from build123d import *

# Parameters (mm, degrees)
F0_R     = 4.1
F1_DEPTH = 10
F2_R     = 10
F3_R     = 2


with BuildPart() as f1:
    # F0 (on Top) → F1 (new body)
    with BuildSketch(Plane.XY):
        Polygon((70, 30), (70, 40), (70, 50), (-8.4782754802, 92.5), (-30, 92.5), (-30, 67.5), (-10, 67.5), (-10, 12.5), (-30, 12.5), (-30, -12.5), (-8.4782754802, -12.5), align=None)
        with Locations((-20, 0)):
            Circle(F0_R, mode=Mode.SUBTRACT)
        with Locations((-20, 80)):
            Circle(F0_R, mode=Mode.SUBTRACT)
        with BuildLine():
            Line((2, 73.1787940384), (52.0543567222, 46.0717998075))
            ThreePointArc((52.0543567222, 46.0717998075), (63.2049623416, 49.472497896), (70, 40))
            ThreePointArc((70, 40), (63.2049623416, 30.527502104), (52.0543567222, 33.9282001925))
            Line((52.0543567222, 33.9282001925), (2, 6.8212059616))
            Line((2, 6.8212059616), (2, 73.1787940384))
        make_face(mode=Mode.SUBTRACT)
        with BuildLine():
            ThreePointArc((56.4697287247, 43.6806500408), (62.0007019388, 44.6911823405), (65.1, 40))
            ThreePointArc((65.1, 40), (62.0007019388, 35.3088176595), (56.4697287247, 36.3193499592))
            Line((56.4697287247, 36.3193499592), (52.0543567222, 33.9282001925))
            ThreePointArc((52.0543567222, 33.9282001925), (63.2049623416, 30.527502104), (70, 40))
            ThreePointArc((70, 40), (63.2049623416, 49.472497896), (52.0543567222, 46.0717998075))
            Line((52.0543567222, 46.0717998075), (56.4697287247, 43.6806500408))
        make_face()
        with BuildLine():
            ThreePointArc((56.4697287247, 36.3193499592), (54.9, 40), (56.4697287247, 43.6806500408))
            Line((56.4697287247, 43.6806500408), (52.0543567222, 46.0717998075))
            ThreePointArc((52.0543567222, 46.0717998075), (50, 40), (52.0543567222, 33.9282001925))
            Line((52.0543567222, 33.9282001925), (56.4697287247, 36.3193499592))
        make_face()
    extrude(amount=F1_DEPTH)

    # F2
    f2_edges = [f1.edges().sort_by_distance(p)[0] for p in [
        (-8.478275, 92.5, 5),
        (-8.478275, -12.5, 5),
        (70, 30, 5),
        (70, 50, 5),
        (52.054357, 46.0718, 5),
        (52.054357, 33.9282, 5),
        (2, 6.821206, 5),
        (2, 73.178794, 5),
    ]]
    fillet(f2_edges, radius=F2_R)

    # F3
    f3_edges = [f1.edges().sort_by_distance(p)[0] for p in [
        (-30, 92.5, 5),
        (-30, 67.5, 5),
        (-30, 12.5, 5),
        (-30, -12.5, 5),
    ]]
    fillet(f3_edges, radius=F3_R)


solid = f1.part
Design review of the part built by this model. Coordinates are the model's own, in mm. A direction names the side the tool comes from. Coordinates: 2 decimals unless noted, no trailing zeros. Order: outer loops, then holes, each group sorted by start corner. A loop starts at its lowest first (then second) coordinate and runs counter-clockwise, first axis right, second up.
Item 1: Take a section at C-C, the plane z = 3.5. Count the separate pieces of the cut face and the enclosed holes in it, then the cut area to 3 significant figures.
Item 2: For pin 1 Ø1 at (y, z) = (21, 2) entering from -X; pin 2 Ø5 at (y, z) = (10, 7.5) entering from +X; pin 3 Ø5 at (y, z) = (33, 4) entering from +X, all flat-tipped, find the tip position at first contact; note any pin that passes through.
Item 3: Take a section at D-D, the plane x = 25.5. Write out the cut boundary in (y, z).
Item 4: The part is to be moulded in two halves that separate along X. For faces 1 (the flat face through (-20, -12.5, 5)), 2 (the cylindrical face through (68.55, 30.77, 5.07)), 3 (the flat face through (30.977, 22.513, 4.93)), 4 (the flat face through (30.58, 57.7, 4.93)), say which applies: pulls with the +X half, pulls with the -X half, needs draft (parallel to the pull), parting line crosses it, or undercut.
Item 5: Take a section at A-A, the plane x = -20. Write out the cut boundary in (y, z), then the cut area to 3 significant figures.
Item 6: For faces 5 (the flat face through (-10, 40, 5)), 6 (the flat face through (-3, 41, 10)), 7 (the cylindrical face through (7.007, 14.945, 5.07)), list the 3-axis set-ups (+Z, -Z, +X, -X, +Y, -Y) from which the entire face can be reached by the end or side of a thin tool; tool diameter is ignored.
Item 7: For line 1 (Y direction, x = -20, z = 5.5); line 2 (Y direction, x = 12.5, z = 7.5); line 3 (X direction, y = 24, z = 1.5), list the stretches that pass through material, from the lowest coordinate up.
Item 8: Take a section at B-B, the plane y = 25.5. Write out the cut boundary in (x, z).
The answers:
1. separate pieces: 1
1. enclosed holes: 4
1. area: 4,060 mm2
2. pin 1: stops at x = -10
2. pin 2: stops at x = 37.69
2. pin 3: stops at x = 69.99
3. outline: (5.9, 0) - (19.55, 0) - (19.55, 10) - (5.9, 10) - close; (60.45, 0) - (74.1, 0) - (74.1, 10) - (60.45, 10) - close
4. face 1: needs draft
4. face 2: pulls with the +X half
4. face 3: undercut
4. face 4: undercut
5. outline: (-12.5, 0) - (-4.1, 0) - (-4.1, 10) - (-12.5, 10) - close; (4.1, 0) - (12.5, 0) - (12.5, 10) - (4.1, 10) - close; (67.5, 0) - (75.9, 0) - (75.9, 10) - (67.5, 10) - close; (84.1, 0) - (92.5, 0) - (92.5, 10) - (84.1, 10) - close
5. area: 336 mm2
6. face 5: +Z, -Z, -X
6. face 6: +Z, +X, -X, +Y, -Y
6. face 7: +Z, -Z
7. line 1: y = -12.5 to -4.1, 4.1 to 12.5, 67.5 to 75.9, 84.1 to 92.5
7. line 2: y = -1.14 to 13.62, 66.38 to 81.14
7. line 3: x = -10 to 2, 33.72 to 58.92
8. outline: (-10, 0) - (2, 0) - (2, 10) - (-10, 10) - close; (36.49, 0) - (61.69, 0) - (61.69, 10) - (36.49, 10) - close
